Read the model definition and answer for the solid it produces. Units are mm, in the model's axes. A direction names the side the tool comes from. Coordinates: 2 decimals unless noted, no trailing zeros. Order: outer loops, then holes, each group sorted by start corner. A loop starts at its lowest first (then second) coordinate and runs counter-clockwise, first axis right, second up.
Autodesk Inventor part; units mm, degrees
ref_plane "YZ Plane" through (0, 0, 0) normal (1, 0, 0) x (0, 1, 0)
ref_plane "XZ Plane" through (0, 0, 0) normal (0, 1, 0) x (-1, 0, 0)
ref_plane "XY Plane" through (0, 0, 0) normal (0, 0, 1) x (1, 0, 0)
sketch "スケッチ1" plane through (0, 0, 0) normal (0, 1, 0) x (-1, 0, 0)
  line L0 (-20, 70) -> (20, 70)
  line L1 (20, 70) -> (20, -70)
  line L2 (20, -70) -> (-20, -70)
  line L3 (-20, -70) -> (-20, 70)
  line L4 (-20, 70) -> (20, -70) construction
  line L5 (20, 70) -> (-20, -70) construction
  point P0 (0, 0)
  dimension "d0" = 140
  dimension "d1" = 40
extrude "プレート1" add sketch "スケッチ1" along normal blind 2.3
sketch "スケッチ2" plane through (17.7, 2.3, 70) normal (1, 0, 0) x (0, 1, 0)
  line L0 (0, -140) -> (0, 0)
  line L1 (0, 0) -> (-12.6, 0)
  line L2 (-12.6, 0) -> (-12.6, -140)
  line L3 (-12.6, -140) -> (0, -140)
edge flange "フランジ1" height 12.6 angle 90 thickness 2.3 bend radius 2.3 thickness toward (1, 0, 0) relief tear relief width 2.3 relief depth 1.15 edges at (20, 0, 0) wall of the first edge with corners at (17.7, 2.3, -70) (17.7, 2.3, 70) (17.7, -10.3, 70) (17.7, -10.3, -70)
bend "曲げ1"
corner "コーナー1"
sketch "スケッチ3" plane through (-17.7, 0, 70) normal (-1, 0, 0) x (0, -1, 0)
  line L0 (0, -140) -> (0, 0)
  line L1 (0, 0) -> (-30, 0)
  line L2 (-30, 0) -> (-30, -140)
  line L3 (-30, -140) -> (0, -140)
edge flange "フランジ2" height 30 angle 90 thickness 2.3 bend radius 2.3 thickness toward (-1, 0, 0) relief tear relief width 2.3 relief depth 1.15 edges at (-20, 2.3, 0) wall of the first edge with corners at (-17.7, 0, -70) (-17.7, 0, 70) (-17.7, 30, 70) (-17.7, 30, -70)
bend "曲げ2"
corner "コーナー2"
sketch "スケッチ4" plane through (20, -10.3, 70) normal (1, 0, 0) x (0, 0, -1)
  line L0 (140, 0) -> (0, 0)
  line L1 (0, 0) -> (0, 8)
  point P0 (70, 10.3)
  point P1 (20, 4)
  point P2 (100, 4)
  dimension "d23" = 4
  dimension "d24" = 80
  dimension "d25" = 20
hole "穴1" at (20, -6.3, 50) at (20, -6.3, -30) direction (-1, 0, 0) diameter 3.2 depth 2.3 tip angle 118
fillet "コーナーR1" radius 4 4 edges at (18.85, -10.3, 70) (18.85, -10.3, -70) (-18.85, 30, -70) (-18.85, 30, 70)
equation "\"d31\" = Thickness"
equation "\"d2\" = Thickness"
equation "\"d3\" = BendReliefWidth"
equation "\"d4\" = BendReliefDepth"
equation "\"d5\" = MinimumRemnant"
equation "\"d6\" = TransitionRadius"
equation "\"d9\" = BendRadius"
equation "\"d10\" = CornerReliefSize"
equation "\"d11\" = GapSize"
equation "\"d12\" = JacobiRadiusSize"
equation "\"d13\" = BendReliefWidth"
equation "\"d14\" = BendReliefDepth"
equation "\"d15\" = MinimumRemnant"
equation "\"d16\" = TransitionRadius"
equation "\"d19\" = BendRadius"
equation "\"d20\" = CornerReliefSize"
equation "\"d21\" = GapSize"
equation "\"d22\" = JacobiRadiusSize"
equation "\"BendRadius\" = Thickness"
equation "\"BendReliefWidth\" = Thickness"
equation "\"BendReliefDepth\" = 0.5 * Thickness"
equation "\"CornerReliefSize\" = 4 * Thickness"
equation "\"MinimumRemnant\" = 2 * Thickness"
equation "\"TransitionRadius\" = BendRadius"
equation "\"JacobiRadiusSize\" = BendRadius"
equation "\"GapSize\" = Thickness"
properties part number "plate7" material "鋼、炭素鋼"
1) Which of the six approach directions +Z, -Z, +X, -X, +Y, -Y give full straight-line access (tool end or side, diameter ignored) to faces 1 (the flat face through (0, 0, 1)), 2 (the cylindrical face through (18.83, -5.33, -28.73)), 3 (the flat face through (-17.7, 17, 1))?
A:
face 1: +Z, -Z, -X, -Y
face 2: +X, -X
face 3: +Z, -Z, +X, +Y
2) A cutting plane is placed at D-D, the plane x = 8.5. Determine the outline of the cut face in (y, z), and give its area (3 significant figures).
A:
outline: (0, -70) - (2.3, -70) - (2.3, 70) - (0, 70) - close
area: 322 mm2
3) Determine the mould class of faces 4 (the flat face through (17.7, -6, 1)), 5 (the cylindrical face through (-18.866, 28.859, -68.797)), 6 (the cylindrical face through (18.83, -5.69, 48.52)) for opening direction Z: pulls with the +Z half, pulls with the -Z half, needs draft (parallel to the pull), parting line crosses it, or undercut.
A:
face 4: needs draft
face 5: pulls with the -Z half
face 6: undercut
4) A cutting plane is placed at B-B, the plane z = 18. Determine the outline of the cut face in (x, y).
A:
outline: (-20, 4.6) arc R4.6 ccw to (-15.4, 0) - (15.4, 0) arc R2.3 cw to (17.7, -2.3) - (17.7, -10.3) - (20, -10.3) - (20, -2.3) arc R4.6 ccw to (15.4, 2.3) - (-15.4, 2.3) arc R2.3 cw to (-17.7, 4.6) - (-17.7, 30) - (-20, 30) - close
5) Flat-ended cylindrical pins translate along their axes: pin 1 Ø3 at (x, z) = (12.5, 31) entering from -Y; pin 2 Ø1 at (x, z) = (4.5, 32) entering from +Y; pin 3 Ø6.5 at (y, z) = (-7.5, 17) entering from -X. Find the tip coordinate at first contact, or state that the pin passes through.
A:
pin 1: stops at y = 0
pin 2: stops at y = 2.3
pin 3: stops at x = 17.7
6) A cutting plane is placed at C-C, the plane y = 23.5. Determine the outline of the cut face in (x, z).
A:
outline: (-20, -70) - (-17.7, -70) - (-17.7, 70) - (-20, 70) - close
7) Straight lines are drawn through the part: line 1 (Z direction, x = 19.5, y = -6.3); line 2 (Y direction, x = 7, z = -52); line 3 (Y direction, x = 19, z = 50). For each, find the intervals that lie inside material, in ascending order.
A:
line 1: z = -70 to -31.6, -28.4 to 48.4, 51.6 to 70
line 2: y = 0 to 2.3
line 3: y = -10.3 to -7.9, -4.7 to 0.56
8) A cutting plane is placed at A-A, the plane z = 50. Determine the outline of the cut face in (x, y), and give its area (3 significant figures).
A:
outline: (-20, 4.6) arc R4.6 ccw to (-15.4, 0) - (15.4, 0) arc R2.3 cw to (17.7, -2.3) - (17.7, -4.7) - (20, -4.7) - (20, -2.3) arc R4.6 ccw to (15.4, 2.3) - (-15.4, 2.3) arc R2.3 cw to (-17.7, 4.6) - (-17.7, 30) - (-20, 30) - close; (17.7, -10.3) - (20, -10.3) - (20, -7.9) - (17.7, -7.9) - close
area: 165 mm2
